from build123d import *

# Parameters (mm, degrees)
F0_R     = 2.5
F0_W     = 40
F0_H     = 40
F0_W_2   = 13.333334
F0_H_2   = 5.842
F0_W_3   = 5.842
F0_H_3   = 20
F1_DEPTH = 5.842


with BuildPart() as f1:
    # F0 (on Front) → F1 (new body)
    with BuildSketch(Plane.XZ):
        Polygon((-25, 55), (-25, 60), (-20, 60), (-20, 65.842), (-30.842, 65.842), (-30.842, 55), align=None)
        Polygon((-20, 60), (-25, 60), (-25, 55), (-25, 50), (-25, 30), (-25, 10), (-25, -10), (-25, -30), (-25, -50), (-25, -55), (-25, -60), (-20, -60), (-6.666667, -60), (6.666667, -60), (20, -60), (25, -60), (25, -55), (25, -50), (25, -30), (25, -10), (25, 10), (25, 30), (25, 50), (25, 55), (25, 60), (20, 60), (6.666667, 60), (-6.666667, 60), align=None)
        with Locations((-7.5, -47.5)):
            Circle(F0_R, mode=Mode.SUBTRACT)
        with Locations((7.5, -47.5)):
            Circle(F0_R, mode=Mode.SUBTRACT)
        with Locations((0, 35)):
            Rectangle(F0_W, F0_H, mode=Mode.SUBTRACT)
        with Locations((0, 62.921)):
            Rectangle(F0_W_2, F0_H_2)
        with Locations((-27.921, 40)):
            Rectangle(F0_W_3, F0_H_3)
        Polygon((20, 65.842), (20, 60), (25, 60), (25, 55), (30.842, 55), (30.842, 65.842), align=None)
        with Locations((-27.921, 0)):
            Rectangle(F0_W_3, F0_H_3)
        with Locations((-27.921, -40)):
            Rectangle(F0_W_3, F0_H_3)
        with Locations((27.921, 40)):
            Rectangle(F0_W_3, F0_H_3)
        Polygon((-25, -60), (-25, -55), (-30.842, -55), (-30.842, -65.842), (-20, -65.842), (-20, -60), align=None)
        with Locations((27.921, 0)):
            Rectangle(F0_W_3, F0_H_3)
        with Locations((27.921, -40)):
            Rectangle(F0_W_3, F0_H_3)
        with Locations((0, -62.921)):
            Rectangle(F0_W_2, F0_H_2)
        Polygon((30.842, -55), (25, -55), (25, -60), (20, -60), (20, -65.842), (30.842, -65.842), align=None)
    extrude(amount=F1_DEPTH)


solid = f1.part
Model file for the job. Use its own axes, mm. A direction names the side the tool comes from. Round coordinates to 2 decimals unless told otherwise and drop trailing zeros. Order: outer loops, then holes, each group sorted by start corner. A loop starts at its lowest first (then second) coordinate and runs counter-clockwise, first axis right, second up. Notation, with made-up numbers: M 86.5,23 L 105.5,23 A13 cw 105.5,34 Z; hole C -36.75,89 d7. An arc over 180 degrees is marked long. Write each question's results on one line, items separated by ' | '. Start each with the question number.
(1) Drop flat-ended pins along their axis: pin 1 (1.5 mm diameter, centred on y = -1.5, z = 52.5, fed in from +X); pin 2 (1.5 mm diameter, centred on x = 13.5, y = -2, fed in from -Z); pin 3 (3 mm diameter, centred on x = 15.5, y = -1, fed in from +Z). Give the stop position or say it passes through.
(2) Saw through at A-A, the plane z = -47.5. Give the cut face in (x, y).
(3) Probe probe 1 along Z at (x, y) = (-7.5, -2.35); probe 2 along Z at (x, y) = (-14.5, -2.5); probe 3 along X at (y, z) = (-1.4, 33.5). List the from-to ranges inside material, lowest first. Write a range as from..to.
(4) Which spindle directions (+Z, -Z, +X, -X, +Y, -Y) get a long thin tool onto all of the face, cutting with end or side? Do faces 4 (the face through (-25, -3, -52)), 5 (the face through (0, -3, 55)), 6 (the face through (13, -3, 60)), 7 (the face through (-20, -3, -63)), 8 (the face through (28, -3, -10)). Say none if no direction does.
(5) Saw through at C-C, the plane x = -17. Give the cut face in (y, z), then the cut area to 3 significant figures.
(6) Two-plate mould, pull along X, no slides. Class faces 1 (the face through (30.842, -3, -40)), 2 (the face through (-8.04, -2.88, -49.94)), 3 (the face through (-30.842, -3, -40)): pulls with the +X half, pulls with the -X half, needs draft (parallel to the pull), parting line crosses it, or undercut.
(7) Saw through at D-D, the plane y = -2.85. State how many separate pieces and enclosed holes the cut face has, then the cut area to 3 significant figures.
(8) Saw through at B-B, the plane x = 2. Give the cut face in (y, z).
Established:
1) pin 1: stops at x = 25 | pin 2: stops at z = -60 | pin 3: stops at z = 60
2) outline: M -30.84,-5.84 L -10,-5.84 L -10,0 L -30.84,0 Z; M -5,-5.84 L 5,-5.84 L 5,0 L -5,0 Z; M 10,-5.84 L 30.84,-5.84 L 30.84,0 L 10,0 Z
3) probe 1: z = -60..-50, -45..15, 55..60 | probe 2: z = -60..15, 55..60 | probe 3: x = -30.84..-20, 20..30.84
4) face 4: -X, +Y, -Y | face 5: +Y, -Y | face 6: +Z, +Y, -Y | face 7: -Z, +Y, -Y | face 8: +X, +Y, -Y
5) outline: M -5.84,-60 L 0,-60 L 0,15 L -5.84,15 Z; M -5.84,55 L 0,55 L 0,60 L -5.84,60 Z | area: 467 mm^2
6) face 1: pulls with the +X half | face 2: undercut | face 3: pulls with the -X half
7) separate pieces: 1 | enclosed holes: 3 | area: 5,590 mm^2
8) outline: M -5.84,-65.84 L 0,-65.84 L 0,15 L -5.84,15 Z; M -5.84,55 L 0,55 L 0,65.84 L -5.84,65.84 Z
